from build123d import *

# Parameters (mm, degrees)
SKETCH1_R           = 5.3578125
BOSS_EXTRUDE1_DEPTH = 3.175


with BuildPart() as part:
    # Sketch1 → Boss-Extrude1 (new body)
    with BuildSketch(Plane.XY):
        Polygon((781.05, 387.35), (-781.05, 387.35), (-781.05, -387.35), (-628.65, -387.35), (-628.65, -342.9), (-501.65, -342.9), (-501.65, -387.35), (501.65, -387.35), (501.65, -342.9), (628.65, -342.9), (628.65, -387.35), (781.05, -387.35), align=None)
        with Locations((-593.725, -44.45)):
            Circle(SKETCH1_R, mode=Mode.SUBTRACT)
        with Locations((-536.575, -44.45)):
            Circle(SKETCH1_R, mode=Mode.SUBTRACT)
        with Locations((536.575, -44.45)):
            Circle(SKETCH1_R, mode=Mode.SUBTRACT)
        with Locations((593.725, -44.45)):
            Circle(SKETCH1_R, mode=Mode.SUBTRACT)
        Polygon((-525.741660624, 69.011766046), (-533.633373454, 78.962186571), (-430.149, 161.036), (-422.25728717, 151.085579476), align=None, mode=Mode.SUBTRACT)
        with Locations((-645.795, 339.09)):
            Circle(SKETCH1_R, mode=Mode.SUBTRACT)
        with Locations((-51.435, 339.459169182)):
            Circle(SKETCH1_R, mode=Mode.SUBTRACT)
        Polygon((533.712268362, 79.061761082), (525.830130005, 69.103754509), (422.266861643, 151.077993427), (430.149, 161.036), align=None, mode=Mode.SUBTRACT)
        with Locations((51.435, 339.338450694)):
            Circle(SKETCH1_R, mode=Mode.SUBTRACT)
        with Locations((645.795, 339.09)):
            Circle(SKETCH1_R, mode=Mode.SUBTRACT)
    extrude(amount=BOSS_EXTRUDE1_DEPTH)


solid = part.part
Part model, mm, in its own coordinate system. A direction names the side the tool comes from. Round coordinates to 2 decimals unless told otherwise and drop trailing zeros. Answer as a JSON object with one key per item and string values.
Item 1: Pull direction X, two halves, no side cores. Call faces 1 (the face through (-482.62, 119.42, 1.57)), 2 (the face through (-11, 5, 0)): pulls with the +X half, pulls with the -X half, needs draft (parallel to the pull), parting line crosses it, or undercut.
Output:
{"face 1": "undercut", "face 2": "needs draft"}
Item 2: Wall check: L1, parallel to X at y = -355, z = 2.45; L2, parallel to X at y = 339.09, z = 2.55; L3, parallel to Y at x = -593.5, z = 2.85. Give the ranges that are in metal, low to high.
Output:
{"L1": "-781.05 to -628.65, -501.65 to 501.65, 628.65 to 781.05", "L2": "-781.05 to -651.15, -640.44 to -56.78, -46.09 to 46.08, 56.79 to 640.44, 651.15 to 781.05", "L3": "-342.9 to -49.8, -39.1 to 387.35"}
Item 3: Tool access for faces 3 (the face through (481.21, 120.62, 1.57)), 4 (the face through (-11, 5, 3.175)): list every direction of +Z, -Z, +X, -X, +Y, -Y with a clear straight run to the whole face (end or side of a thin tool).
Output:
{"face 3": "+Z, -Z", "face 4": "+Z, +X, -X, +Y, -Y"}
Item 4: Pin check, flat tips, straight feed: pin 1 (8.5 mm diameter, centred on x = 593.725, y = -44.45, fed in from -Z); pin 2 (1 mm diameter, centred on x = -520, z = 1.5, fed in from -Y). Stop position of each tip, or through.
Output:
{"pin 1": "through", "pin 2": "y = -342.9"}
